Geometry: final body of the model. Coordinates: model frame, mm. A direction names the side the tool comes from. Coordinates: 2 decimals unless noted, no trailing zeros. Order: outer loops, then holes, each group sorted by start corner. A loop starts at its lowest first (then second) coordinate and runs counter-clockwise, first axis right, second up. Notation, with made-up numbers: (86, 60.25) -> (139, 60.25) arc R21 ccw to (139, 94.25) -> close; hole circle Ø11 at (17, -10). An arc over 180 degrees is marked (long way). Answer in a Markdown table with one row per item. Add a question column.
1) Section query A-A on y = 15. Return the cut outline in (x, z), then the cut area to 3 significant figures.
2) Ray query, line 1 (Y direction, x = 13, z = -5); line 2 (Z direction, x = 20.5, y = 18.5); line 3 (X direction, y = 9.5, z = -46.5). Return the intervals inside material, ascending. Write a range as from..to.
3) Contact query for flat-ended pins moving along their axis: P1, Ø1, axis at y = 3.5, z = 9, coming from the -X side; P2, Ø2, axis at x = 32.5, z = 19.5, coming from the -Y side; P3, Ø2, axis at y = 17, z = -43, coming from the -X side; P4, Ø6, axis at y = 12, z = 27, coming from the -X side. Output: stop coordinate, or through.
4) Pull-direction query (Z, two-part tool) for faces 1 (the face through (-10, 14, -35)), 2 (the face through (34, 14, 10)); classes: +Z half, -Z half, draft (parallel to the pull), parting line (faces both ways), or undercut.
5) Set-up query: faces 3 (the face through (-34, 14, -10)), 4 (the face through (10, 14, -34)), 5 (the face through (-29, 20, 29)). Return all of +Z, -Z, +X, -X, +Y, -Y with unobstructed straight access to the full face (end or side cutting, diameter ignored); none if empty.
6) Section query B-B on z = 21. Return the cut outline in (x, y).
7) Section query C-C on x = -39.5. Return the cut outline in (y, z).
```python
from build123d import *

# Parameters (mm, degrees)
BOSS_EXTRUDE1_DEPTH = 20
CUT_EXTRUDE1_START  = 8
CUT_EXTRUDE1_DEPTH  = 12


with BuildPart() as part:
    # Sketch1 → Boss-Extrude1 (new body)
    with BuildSketch(Plane(origin=(0, 0, 0), x_dir=(1, 0, 0), z_dir=(0, 1, 0))):
        with BuildLine():
            Line((-59.160797831, 10), (-10, 10))
            Line((-10, 10), (-10, 59.160797831))
            ThreePointArc((-10, 59.160797831), (-42.426406871, 42.426406871), (-59.160797831, 10))
        make_face()
        with BuildLine():
            Line((-10, 59.160797831), (-10, 10))
            Line((-10, 10), (-59.160797831, 10))
            ThreePointArc((-59.160797831, 10), (-60, 0), (-59.160797831, -10))
            Line((-59.160797831, -10), (-10, -10))
            Line((-10, -10), (-10, -59.160797831))
            ThreePointArc((-10, -59.160797831), (0, -60), (10, -59.160797831))
            Line((10, -59.160797831), (10, -10))
            Line((10, -10), (59.160797831, -10))
            ThreePointArc((59.160797831, -10), (59.789831367, -5.017575617), (60, 0))
            ThreePointArc((60, 0), (59.789831367, 5.017575617), (59.160797831, 10))
            Line((59.160797831, 10), (10, 10))
            Line((10, 10), (10, 59.160797831))
            ThreePointArc((10, 59.160797831), (0, 60), (-10, 59.160797831))
        make_face()
        with BuildLine():
            Line((-10, -10), (-59.160797831, -10))
            ThreePointArc((-59.160797831, -10), (-42.426406871, -42.426406871), (-10, -59.160797831))
            Line((-10, -59.160797831), (-10, -10))
        make_face()
        with BuildLine():
            ThreePointArc((59.160797831, 10), (42.426406871, 42.426406871), (10, 59.160797831))
            Line((10, 59.160797831), (10, 10))
            Line((10, 10), (59.160797831, 10))
        make_face()
        with BuildLine():
            Line((10, -10), (10, -59.160797831))
            ThreePointArc((10, -59.160797831), (42.426406871, -42.426406871), (59.160797831, -10))
            Line((59.160797831, -10), (10, -10))
        make_face()
    extrude(amount=BOSS_EXTRUDE1_DEPTH)

    # Sketch1<3> → Cut-Extrude1 (cut)
    with BuildSketch(Plane(origin=(0, 0, 0), x_dir=(1, 0, 0), z_dir=(0, 1, 0)).offset(CUT_EXTRUDE1_START)):
        with BuildLine():
            Line((-10, 59.160797831), (-10, 10))
            Line((-10, 10), (-59.160797831, 10))
            ThreePointArc((-59.160797831, 10), (-60, 0), (-59.160797831, -10))
            Line((-59.160797831, -10), (-10, -10))
            Line((-10, -10), (-10, -59.160797831))
            ThreePointArc((-10, -59.160797831), (0, -60), (10, -59.160797831))
            Line((10, -59.160797831), (10, -10))
            Line((10, -10), (59.160797831, -10))
            ThreePointArc((59.160797831, -10), (59.789831367, -5.017575617), (60, 0))
            ThreePointArc((60, 0), (59.789831367, 5.017575617), (59.160797831, 10))
            Line((59.160797831, 10), (10, 10))
            Line((10, 10), (10, 59.160797831))
            ThreePointArc((10, 59.160797831), (0, 60), (-10, 59.160797831))
        make_face()
    extrude(amount=CUT_EXTRUDE1_DEPTH, mode=Mode.SUBTRACT)


solid = part.part
```
Result:
| question | item | result |
|---|---|---|
| 1 | outline | (-59.16, -10) arc R60 ccw to (-10, -59.16) -> (-10, -10) -> close; (-59.16, 10) -> (-10, 10) -> (-10, 59.16) arc R60 ccw to start; (10, -59.16) arc R60 ccw to (59.16, -10) -> (10, -10) -> close; (10, 10) -> (59.16, 10) arc R60 ccw to (10, 59.16) -> close |
| 1 | area | 6,930 mm2 |
| 2 | line 1 | 0..8 |
| 2 | line 2 | -56.39..-10, 10..56.39 |
| 2 | line 3 | -37.92..-10, 10..37.92 |
| 3 | P1 | x = -59.39 |
| 3 | P2 | y = 0 |
| 3 | P3 | x = -42.85 |
| 3 | P4 | x = -54.99 |
| 4 | face 1 | draft |
| 4 | face 2 | undercut |
| 5 | face 3 | +X, -X, +Y |
| 5 | face 4 | +Z, -Z, +Y |
| 5 | face 5 | +Z, -Z, +X, -X, +Y |
| 6 | outline | (-56.2, 0) -> (56.2, 0) -> (56.2, 20) -> (10, 20) -> (10, 8) -> (-10, 8) -> (-10, 20) -> (-56.2, 20) -> close |
| 7 | outline | (0, -45.16) -> (20, -45.16) -> (20, -10) -> (8, -10) -> (8, 10) -> (20, 10) -> (20, 45.16) -> (0, 45.16) -> close |
